```python
from build123d import *

# Parameters (mm, degrees)
SKETCH1_W            = 29.5
SKETCH1_H            = 6.75
BOSS_EXTRUDE10_DEPTH = 3.5
BOSS_EXTRUDE15_DEPTH = 1.25
SKETCH1_17_W         = 34.75
SKETCH1_17_H         = 2.924143722
BOSS_EXTRUDE17_DEPTH = 30.75
BOSS_EXTRUDE18_DEPTH = 1.25
SKETCH2_9_R          = 1.75
BOSS_EXTRUDE19_DEPTH = 1.75
BOSS_EXTRUDE19_TAPER = 4
FILLET1_R            = 2
FILLET2_R            = 4
CUT_EXTRUDE1_START   = -2.25
SKETCH3_W            = 5.75
SKETCH3_H            = 1.125
CUT_EXTRUDE1_DEPTH   = 2.25


with BuildPart() as part:
    # Sketch1 → Boss-Extrude10 (new body)
    with BuildSketch(Plane.XY):
        with Locations((0, 3.375)):
            Rectangle(SKETCH1_W, SKETCH1_H)
        with BuildLine():
            Line((-12.265078429, 5.016721387), (0, 6.25))
            Line((0, 6.25), (12.265078429, 5.016721387))
            ThreePointArc((12.265078429, 5.016721387), (13.75, 3.375), (12.265078429, 1.733278613))
            Line((12.265078429, 1.733278613), (0, 0.5))
            Line((0, 0.5), (-12.265078429, 1.733278613))
            ThreePointArc((-12.265078429, 1.733278613), (-13.75, 3.375), (-12.265078429, 5.016721387))
        make_face(mode=Mode.SUBTRACT)
    extrude(amount=BOSS_EXTRUDE10_DEPTH)

    # Sketch1<16> → Boss-Extrude15 (add)
    with BuildSketch(Plane.XY):
        with BuildLine():
            ThreePointArc((-12.265078429, 5.016721387), (-13.75, 3.375), (-12.265078429, 1.733278613))
            Line((-12.265078429, 1.733278613), (0, 0.5))
            Line((0, 0.5), (12.265078429, 1.733278613))
            ThreePointArc((12.265078429, 1.733278613), (13.75, 3.375), (12.265078429, 5.016721387))
            Line((12.265078429, 5.016721387), (0, 6.25))
            Line((0, 6.25), (-12.265078429, 5.016721387))
        make_face()
    extrude(amount=BOSS_EXTRUDE15_DEPTH)

    # Sketch1<17> → Boss-Extrude17 (add)
    with BuildSketch(Plane.XY):
        with Locations((32.125, 3.375)):
            Rectangle(SKETCH1_17_W, SKETCH1_17_H)
    extrude(amount=BOSS_EXTRUDE17_DEPTH)

    # Sketch2 → Boss-Extrude18 (add)
    with BuildSketch(Plane.XY.offset(30.75)):
        Polygon((13.5, 5.875), (-8.061356684, 5.875), (-8.061356684, 0.875), (14.75, 0.875), (14.75, 5.875), align=None)
    extrude(amount=-BOSS_EXTRUDE18_DEPTH)

    # Sketch2<9> → Boss-Extrude19 (add)
    with BuildSketch(Plane.XY.offset(30.75)):
        with Locations((0, 3.375)):
            Circle(SKETCH2_9_R)
    extrude(amount=BOSS_EXTRUDE19_DEPTH, taper=BOSS_EXTRUDE19_TAPER)

    # Fillet1
    # the kernel refuses this fillet: 2 mm, written as the material it adds along each edge
    with BuildSketch(Plane(origin=(14.75, 1.912928139, 0), x_dir=(0, -1, 0), z_dir=(0, 0, 1))) as fillet1_piece_1:
        with BuildLine():
            CenterArc((2, 1.998103724), FILLET1_R, 180, 87.504786267)
            Line((0, 1.998103724), (0, 0))
            Line((0, 0), (1.912928139, 0))
        make_face()
    extrude(amount=3.5)
    with BuildSketch(Plane(origin=(14.75, 4.837071861, 0), x_dir=(1, 0, 0), z_dir=(0, 0, 1))) as fillet1_piece_2:
        with BuildLine():
            CenterArc((1.998103724, 2), FILLET1_R, 182.495213733, 87.504786267)
            Line((0, 1.912928139), (0, 0))
            Line((0, 0), (1.998103724, 0))
        make_face()
    extrude(amount=3.5)
    with BuildSketch(Plane(origin=(14.75, 1.912928139, 29.5), x_dir=(1, 0, 0), z_dir=(0, 0, 1))) as fillet1_piece_3:
        with BuildLine():
            CenterArc((1.753401761, -2), FILLET1_R, 90, 61.246917848)
            Line((0, -1.037928139), (0, 0))
            Line((0, 0), (1.753401761, 0))
        make_face()
    extrude(amount=1.25)
    with BuildSketch(Plane(origin=(14.75, 4.837071861, 29.5), x_dir=(1, 0, 0), z_dir=(0, 0, 1))) as fillet1_piece_4:
        with BuildLine():
            CenterArc((1.753401761, 2), FILLET1_R, 208.753082152, 61.246917848)
            Line((0, 1.037928139), (0, 0))
            Line((0, 0), (1.753401761, 0))
        make_face()
    extrude(amount=1.25)

    # Fillet2
    # the kernel refuses this fillet: 4 mm, written as the material it takes off along each edge
    with BuildSketch(Plane(origin=(-14.75, 6.75, -10), x_dir=(0, -1, 0), z_dir=(0, 0, 1)), Plane(origin=(-14.75, 0, -10), x_dir=(1, 0, 0), z_dir=(0, 0, 1))) as fillet2_piece_1:
        with BuildLine():
            CenterArc((FILLET2_R, FILLET2_R), FILLET2_R, 180, 90)
            Line((0, FILLET2_R), (0, 0))
            Line((0, 0), (FILLET2_R, 0))
        make_face()
    extrude(amount=23.5, mode=Mode.SUBTRACT)

    # Sketch3 → Cut-Extrude1 (cut)
    with BuildSketch(Plane.XY.offset(3.5).offset(CUT_EXTRUDE1_START)):
        with Locations((-0.102107464, 6.1875)):
            Rectangle(SKETCH3_W, SKETCH3_H)
        with Locations((-0.102107464, 0.5625)):
            Rectangle(SKETCH3_W, SKETCH3_H)
    extrude(amount=CUT_EXTRUDE1_DEPTH, mode=Mode.SUBTRACT)


solid = part.part
```
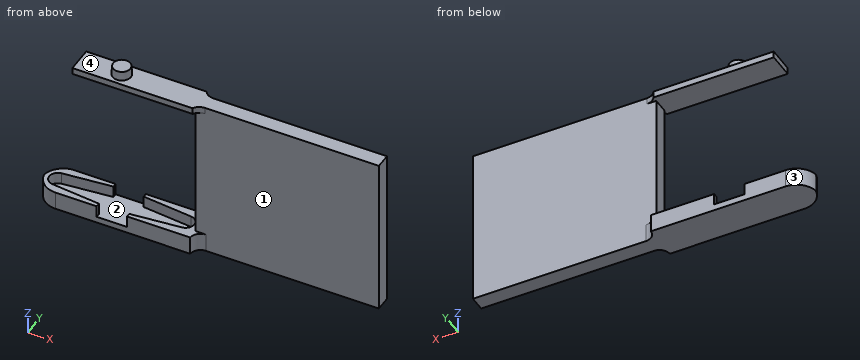
CAD build for the part. Positions are in the model's coordinates, mm. Face numbers are marked on the shaded views. Round coordinates to 2 decimals unless told otherwise and drop trailing zeros. Order: outer loops, then holes, each group sorted by start corner. A loop starts at its lowest first (then second) coordinate and runs counter-clockwise, first axis right, second up.
Item 1: Saw through at A-A on x = 0. Write the cut outline in (y, z) (3 decimals).
Item 2: Mould opens along Y. For the marked faces 1, 2, 3 and 4 say: pulls with the +Y half, pulls with the -Y half, needs draft (parallel to the pull), parting line crosses it, or undercut.
Item 3: Saw through at C-C on z = 10. Write the cut outline in (x, y), then the cut area to 3 significant figures.
Item 4: Pin check, flat tips, straight feed: pin 1 (4 mm diameter, centred on y = 1, z = 8, fed in from +X); pin 2 (0.9 mm diameter, centred on y = 0.5, z = 2, fed in from -X); pin 3 (3 mm diameter, centred on x = 10, y = 4.5, fed in from +Z); pin 4 (0.6 mm diameter, centred on x = 4.5, z = 30.5, fed in from +Y) (3 decimals). Stop position of each tip, or through.
Item 5: Saw through at B-B on x = -7. Write the cut outline in (y, z) (3 decimals), then the cut area to 3 significant figures.
Item 6: Probe line 1 along Z through (x, y) = (-2.5, 5); line 2 along Z through (x, y) = (35, 2); line 3 along X through (y, z) = (3.75, 11.5). List the from-to ranges inside material, lowest first.
Reported:
1. outline: (0, 0) - (6.75, 0) - (6.75, 1.25) - (0, 1.25) - close; (0.875, 29.5) - (5.875, 29.5) - (5.875, 30.75) - (5.125, 30.75) - (5.003, 32.5) - (1.747, 32.5) - (1.625, 30.75) - (0.875, 30.75) - close
2. face 1: pulls with the -Y half
2. face 2: undercut
2. face 3: pulls with the +Y half
2. face 4: needs draft
3. outline: (14.75, 1.91) - (49.5, 1.91) - (49.5, 4.84) - (14.75, 4.84) - close
3. area: 102 mm2
4. pin 1: stops at x = 49.5
4. pin 2: stops at x = -13.34
4. pin 3: stops at z = 30.75
4. pin 4: stops at y = 5.875
5. outline: (0, 0) - (6.75, 0) - (6.75, 3.5) - (5.546, 3.5) - (5.546, 1.25) - (1.204, 1.25) - (1.204, 3.5) - (0, 3.5) - close; (0.875, 29.5) - (5.875, 29.5) - (5.875, 30.75) - (0.875, 30.75) - close
5. area: 20.1 mm2
6. line 1: z = 0 to 1.25, 29.5 to 30.75
6. line 2: z = 0 to 30.75
6. line 3: x = 14.75 to 49.5
